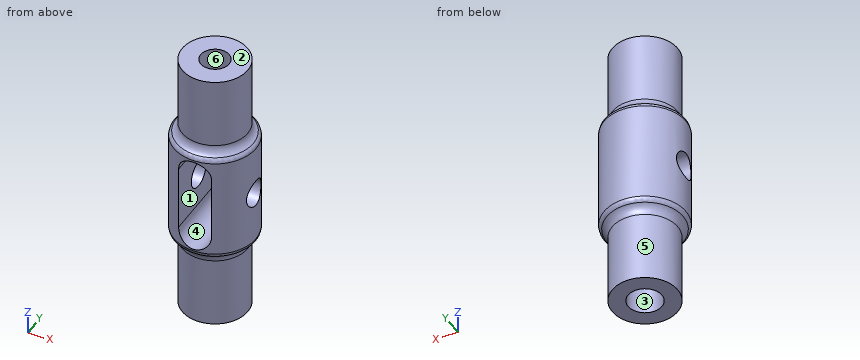
```python
from build123d import *

# Parameters (mm, degrees)
SKETCH1_R           = 6
BOSS_EXTRUDE1_DEPTH = 7.5
SKETCH2_R           = 7.5
BOSS_EXTRUDE2_DEPTH = 20
SKETCH3_R           = 3.1
CUT_EXTRUDE1_DEPTH  = 15
SKETCH4_R           = 2.5
CUT_EXTRUDE2_DEPTH  = 11
CUT_EXTRUDE3_DEPTH  = 20
FILLET1_R           = 2
FILLET2_R           = 1
SKETCH7_R           = 2.6
CUT_EXTRUDE4_DEPTH  = 15
CUT_EXTRUDE5_START  = -6
CUT_EXTRUDE5_DEPTH  = 6


with BuildPart() as part:
    # Sketch1 → Boss-Extrude1 (new, symmetric)
    with BuildSketch(Plane.XY):
        Circle(SKETCH1_R)
    boss_extrude1 = extrude(amount=BOSS_EXTRUDE1_DEPTH, both=True)

    # Sketch2 → Boss-Extrude2 (add)
    with BuildSketch(Plane.XY.offset(7.5)):
        Circle(SKETCH2_R)
    extrude(amount=BOSS_EXTRUDE2_DEPTH)

    # Mirror1: Boss-Extrude1 across plane
    add(boss_extrude1.mirror(Plane.XY.offset(17.5)))

    # Sketch3 → Cut-Extrude1 (cut)
    with BuildSketch(Plane(origin=(0, 0, -7.5), x_dir=(-1, 0, 0), z_dir=(0, 0, -1))):
        Circle(SKETCH3_R)
    extrude(amount=-CUT_EXTRUDE1_DEPTH, mode=Mode.SUBTRACT)

    # Sketch4 → Cut-Extrude2 (cut, symmetric)
    with BuildSketch(Plane(origin=(0, 0, 0), x_dir=(0, 0, -1), z_dir=(1, 0, 0))):
        with Locations(Location((-17.655484387, 0, 0), (0, 0, 180))):
            Circle(SKETCH4_R)
    extrude(amount=CUT_EXTRUDE2_DEPTH, both=True, mode=Mode.SUBTRACT)

    # Sketch6 → Cut-Extrude3 (cut)
    with BuildSketch(Plane(origin=(0, 0, 0), x_dir=(1, 0, 0), z_dir=(0, 1, 0))):
        with BuildLine():
            Line((3, -11.5), (3, -23.5))
            ThreePointArc((3, -23.5), (0, -26.5), (-3, -23.5))
            Line((-3, -23.5), (-3, -11.5))
            ThreePointArc((-3, -11.5), (0, -8.5), (3, -11.5))
        make_face()
    extrude(amount=-CUT_EXTRUDE3_DEPTH, mode=Mode.SUBTRACT)

    # Fillet1
    # the kernel refuses this fillet: 2 mm, written as the material it adds along each edge
    with BuildSketch(Plane(origin=(0, 0, 7.5), x_dir=(1, 0, 0), z_dir=(0, -1, 0))) as fillet1_piece_1:
        with BuildLine():
            CenterArc((8, -1.936491673), FILLET1_R, 104.477512186, 75.522487814)
            Line((6, -1.936491673), (5.96, -1.936491673))
            Line((5.96, -1.936491673), (5.96, 0))
            Line((5.96, 0), (6, 0.04))
            ThreePointArc((6, 0.04), (6.75, 0.04), (7.49, 0.038729833))
            Line((7.49, 0.038729833), (7.5, 0))
        make_face()
    revolve(axis=Axis((0, 0, 7.5), (0, 0, 1)))
    with BuildSketch(Plane(origin=(0, 0, 27.5), x_dir=(1, 0, 0), z_dir=(0, -1, 0))) as fillet1_piece_2:
        with BuildLine():
            CenterArc((8, 1.936491673), FILLET1_R, 180, 75.522487814)
            Line((6, 1.936491673), (5.96, 1.936491673))
            Line((5.96, 1.936491673), (5.96, 0))
            Line((5.96, 0), (6, -0.04))
            ThreePointArc((6, -0.04), (6.75, -0.04), (7.49, -0.038729833))
            Line((7.49, -0.038729833), (7.5, 0))
        make_face()
    revolve(axis=Axis((0, 0, 27.5), (0, 0, 1)))

    # Fillet2
    fillet2_edges = [part.edges().sort_by_distance(p)[0] for p in [
        (-7.5, 0, 7.5),
        (-7.5, 0, 27.5),
    ]]
    fillet(fillet2_edges, radius=FILLET2_R)

    # Sketch7 → Cut-Extrude4 (cut)
    with BuildSketch(Plane.XY.offset(42.5)):
        Circle(SKETCH7_R)
    extrude(amount=-CUT_EXTRUDE4_DEPTH, mode=Mode.SUBTRACT)

    # Sketch8 → Cut-Extrude5 (cut)
    with BuildSketch(Plane.XZ.offset(CUT_EXTRUDE5_START)):
        with BuildLine():
            Line((3, 20.155484387), (-3, 20.155484387))
            Line((-3, 20.155484387), (-3, 15.155484387))
            Line((-3, 15.155484387), (-3, 11.5))
            ThreePointArc((-3, 11.5), (0, 8.5), (3, 11.5))
            Line((3, 11.5), (3, 15.155484387))
            Line((3, 15.155484387), (3, 20.155484387))
        make_face()
        with BuildLine():
            Line((-3, 20.155484387), (3, 20.155484387))
            Line((3, 20.155484387), (3, 23.5))
            ThreePointArc((3, 23.5), (0, 26.5), (-3, 23.5))
            Line((-3, 23.5), (-3, 20.155484387))
        make_face()
    extrude(amount=CUT_EXTRUDE5_DEPTH, mode=Mode.SUBTRACT)


solid = part.part
```
Here's how the part is built. I have some questions about the finished solid (model axes, mm). Face numbers are marked on the shaded views. A direction names the side the tool comes from. Give positions to 0.01 mm unless a question says otherwise; leave off trailing zeros. Order: outer loops, then holes, each group sorted by start corner. A loop starts at its lowest first (then second) coordinate and runs counter-clockwise, first axis right, second up. Notation, with made-up numbers: (-18.5, -26) - (35.5, -26) arc R30 cw to (35.5, 5) - close; hole circle Ø7 at (-24.5, -24). An arc over 180 degrees is marked (long way). Answer as a JSON object with one key per item and string values. Group by question number.
Item 1: If we section it at B-B on z = -4: Please give me the cut outline in (x, y).
Item 2: Which directions (+Z, -Z, +X, -X, +Y, -Y) give clear straight access to the entire face, cutting with the end or side of a thin tool? Please do the marked faces 4, 5 and 6.
Item 3: If we section it at A-A on z = 32.5: Please give me the cut outline in (x, y).
Item 4: Please list where these lines run through material, in increasing order: probe 1 along Y at (x, z) = (0, 38.5); probe 2 along X at (y, z) = (0.5, 14); probe 3 along Z at (x, y) = (1.5, -5.5).
Item 5: If we mould it in two halves opening along Z, with no side actions, what happens to the marked faces 1, 2 and 3? For each: pulls with the +Z half, pulls with the -Z half, needs draft (parallel to the pull), parting line crosses it, or undercut.
Item 6: For P1, Ø6, axis at x = 0, y = 0, coming from the -Z side; P2, Ø1.5, axis at x = -5, z = 13, coming from the -Y side; P3, Ø3, axis at x = -5, z = -1.5, coming from the -Y side; P4, Ø4.5, axis at y = 0, z = 17.66, coming from the -X side, each with a flat end and sliding along its axis, tell me the tip position at first contact or that it passes through.
Result set:
{
 "1": {"outline": "circle Ø12 at (0, 0); hole circle Ø6.2 at (0, 0)"},
 "2": {"face 4": "-Y", "face 5": "-Z", "face 6": "+Z"},
 "3": {"outline": "circle Ø12 at (0, 0); hole circle Ø5.2 at (0, 0)"},
 "4": {"probe 1": "-6 to -2.6, 2.6 to 6", "probe 2": "-7.48 to -3, 3 to 7.48", "probe 3": "-7.5 to 8.9, 26.1 to 42.5"},
 "5": {"face 1": "undercut", "face 2": "pulls with the +Z half", "face 3": "needs draft"},
 "6": {"P1": "z = 7.5", "P2": "y = -6.18", "P3": "y = -4.87", "P4": "through"}
}
